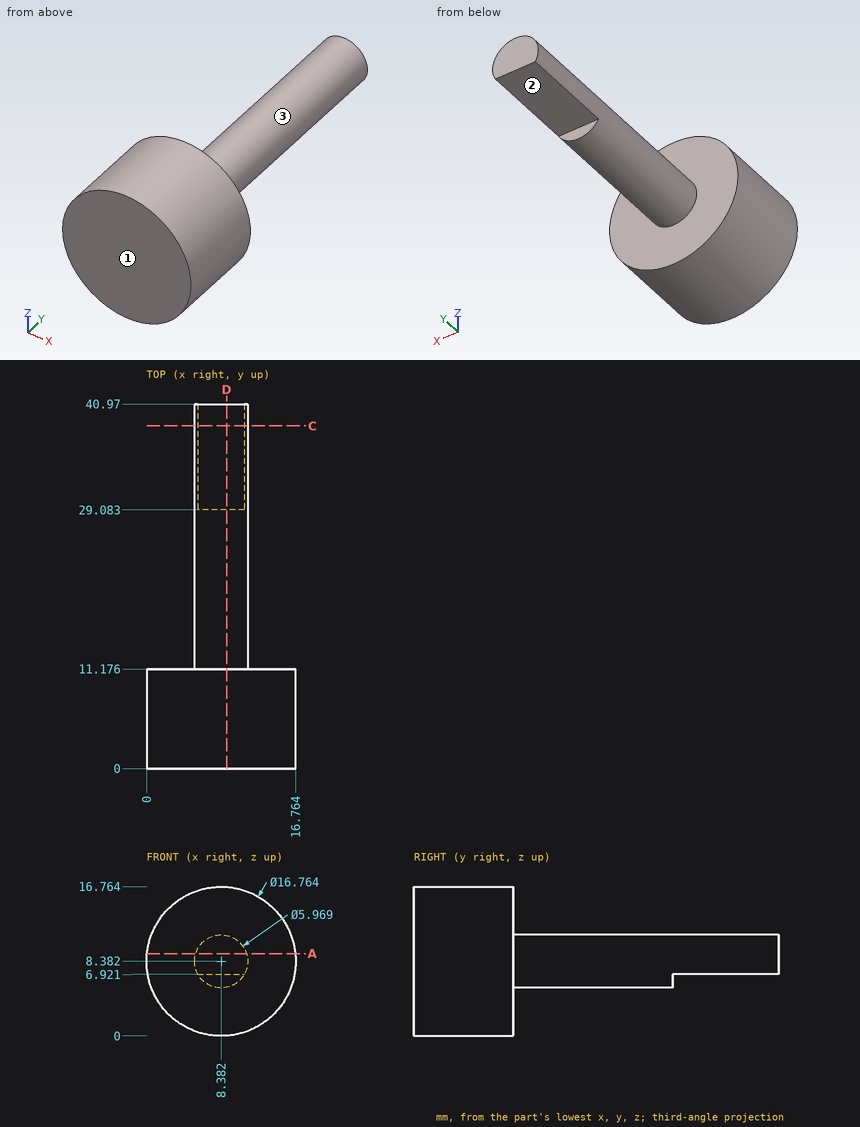
Answer from the drawing. Dimensions are ordinates in mm from the lowest x, y and z of the part. A direction names the side the tool comes from. Coordinates: 2 decimals unless noted, no trailing zeros. Write each loop counter-clockwise with the first axis right and the second up, starting at its lowest first coordinate (ties: lowest second). Pieces come first, ordered by that corner, then holes. Notation, with made-up numbers: (-11.75, 13.25) - (26.25, 13.25) arc R21 ccw to (26.25, 29.25) - close; hole circle Ø11 at (-16, -12). An arc over 180 degrees is marked (long way). Return JSON: item names as keys, results as strings.
1. Consider line 1 along Y through (x, z) = (14.5, 7.25) (1 decimal); line 2 along X through (y, z) = (29, 8.5) (1 decimal); line 3 along Z through (x, y) = (7.25, 24.5) (1 decimal). Determine where each line is inside the solid, lowest interval first.
Final values:
{"line 1": "0 to 11.2", "line 2": "5.4 to 11.4", "line 3": "5.6 to 11.1"}
2. Which of the six approach directions +Z, -Z, +X, -X, +Y, -Y give full straight-line access (tool end or side, diameter ignored) to the marked faces 1, 2 and 3?
Final values:
{"face 1": "+Z, -Z, +X, -X, -Y", "face 2": "-Z, +X, -X, +Y", "face 3": "+Y"}
3. The part is cut by section D-D on x = 9. Determine the outline of the cut face in (y, z) (1 decimal).
Final values:
{"outline": "(0, 0) - (11.2, 0) - (11.2, 5.5) - (29.1, 5.5) - (29.1, 6.9) - (41, 6.9) - (41, 11.3) - (11.2, 11.3) - (11.2, 16.7) - (0, 16.7) - close"}
4. Each of these flat-tipped pins is pushed along its axis until it touches: pin 1 Ø5.5 at (x, y) = (8, 33.5) entering from -Z; pin 2 Ø4 at (x, y) = (7, 32.5) entering from +Z; pin 3 Ø10 at (y, z) = (24.5, 8.5) entering from -X. Where does it stop, or does it pass through?
Final values:
{"pin 1": "z = 6.92", "pin 2": "z = 11.37", "pin 3": "x = 5.4"}
5. The part is cut by section C-C on y = 38.5. Determine the outline of the cut face in (x, z) (1 decimal).
Final values:
{"outline": "(5.8, 6.9) - (11, 6.9) arc R3 ccw (long way) to start"}
6. The part is cut by section A-A on z = 9.25. Determine the outline of the cut face in (x, y) (1 decimal).
Final values:
{"outline": "(0, 0) - (16.7, 0) - (16.7, 11.2) - (11.2, 11.2) - (11.2, 41) - (5.5, 41) - (5.5, 11.2) - (0, 11.2) - close"}
